Part model, mm, in its own coordinate system. Face numbers are marked on the shaded views. A direction names the side the tool comes from. Round coordinates to 2 decimals unless told otherwise and drop trailing zeros. Loops run counter-clockwise (first coordinate to the right, second up) from the corner with the lowest first, then second, coordinate; pieces in that order, holes last. Notation, with made-up numbers: (33, 40) - (65, 40) arc R23 cw to (65, 76) - close; hole circle Ø5 at (20.5, -15.75). An arc over 180 degrees is marked (long way). Write each question's results on one line, items separated by ' | '. Start each with the question number.
(1) Cut at D-D, the plane x = -32. List the corners of the cut face in (y, z).
(2) Cut at B-B, the plane x = -56. List the corners of the cut face in (y, z).
(3) Flat gauge pins, fed straight in: P1, Ø3, axis at x = -71.55, z = -24.85, coming from the +Y side; P2, Ø2, axis at y = -43.5, z = -5, coming from the +X side; P3, Ø1.5, axis at y = -50.5, z = 24, coming from the +X side; P4, Ø6, axis at x = 71.55, z = -24.85, coming from the +Y side. Where does each tip first touch, or does it go through?
(4) Cut at C-C, the plane z = -17. List the corners of the cut face in (x, y).
(5) Tool access for the marked faces 4, 5, 6 and 7: list every direction of +Z, -Z, +X, -X, +Y, -Y with a clear straight run to the whole face (end or side of a thin tool).
(6) Cut at A-A, the plane x = 31.75. List the corners of the cut face in (y, z), then the cut area to 3 significant figures.
(7) Drill centre lines: L1, parallel to Z at x = 31.75, y = -0.4; L2, parallel to Z at x = -39, y = -20; L3, parallel to Z at x = -31, y = -4.5. Where is each one in solid material? Low to high.
(8) Mould opens along Z. For the marked faces 1, 2 and 3 say: released by +Z, released by -Z, zero draft, split by the parting line, or undercut.
from build123d import *

# Parameters (mm, degrees)
SKETCH1_W             = 171.0436
SKETCH1_H             = 78.613
BOSS_EXTRUDE1_DEPTH   = 58.42
CUT_EXTRUDE1_DEPTH    = 45.72
BOSS_EXTRUDE2_DEPTH   = 7.62
FILLET1_R             = 25.4
F_6_CLEARANCE_HOLE2_D = 3.7973
SKETCH12_R            = 3.302
CUT_EXTRUDE2_DEPTH    = 0.889


with BuildPart() as part:
    # Sketch1 → Boss-Extrude1 (new body)
    with BuildSketch(Plane.XZ):
        with Locations((0, 0.485871825)):
            Rectangle(SKETCH1_W, SKETCH1_H)
        with BuildLine():
            Line((-73.683610441, -1.938038616), (-48.639210441, -26.982438616))
            ThreePointArc((-48.639210441, -26.982438616), (-43.966930256, -30.104356426), (-38.4556, -31.200628175))
            Line((-38.4556, -31.200628175), (38.4556, -31.200628175))
            ThreePointArc((38.4556, -31.200628175), (43.966930256, -30.104356426), (48.639210441, -26.982438616))
            Line((48.639210441, -26.982438616), (73.683610441, -1.938038616))
            ThreePointArc((73.683610441, -1.938038616), (76.805528251, 13.756902081), (63.5, 22.647371825))
            Line((63.5, 22.647371825), (-63.5, 22.647371825))
            ThreePointArc((-63.5, 22.647371825), (-76.805528251, 13.756902081), (-73.683610441, -1.938038616))
        make_face(mode=Mode.SUBTRACT)
    extrude(amount=BOSS_EXTRUDE1_DEPTH)

    # Sketch2 → Cut-Extrude1 (cut)
    with BuildSketch(Plane.XZ.offset(58.42)):
        with BuildLine():
            ThreePointArc((54.027364114, -32.370592289), (46.882978011, -37.144318464), (38.4556, -38.820628175))
            Line((38.4556, -38.820628175), (85.5218, -38.820628175))
            Line((85.5218, -38.820628175), (85.5218, 8.245571825))
            ThreePointArc((85.5218, 8.245571825), (83.845490289, -0.181806186), (79.071764114, -7.326192289))
            Line((79.071764114, -7.326192289), (54.027364114, -32.370592289))
        make_face()
        with BuildLine():
            Line((-85.5218, 8.245571825), (-85.5218, -38.820628175))
            Line((-85.5218, -38.820628175), (-38.4556, -38.820628175))
            ThreePointArc((-38.4556, -38.820628175), (-46.882978011, -37.144318464), (-54.027364114, -32.370592289))
            Line((-54.027364114, -32.370592289), (-79.071764114, -7.326192289))
            ThreePointArc((-79.071764114, -7.326192289), (-83.845490289, -0.181806186), (-85.5218, 8.245571825))
        make_face()
        with BuildLine():
            Line((-85.5218, 39.792371825), (-85.5218, 8.245571825))
            ThreePointArc((-85.5218, 8.245571825), (-79.071764114, 23.817335939), (-63.5, 30.267371825))
            Line((-63.5, 30.267371825), (63.5, 30.267371825))
            ThreePointArc((63.5, 30.267371825), (79.071764114, 23.817335939), (85.5218, 8.245571825))
            Line((85.5218, 8.245571825), (85.5218, 39.792371825))
            Line((85.5218, 39.792371825), (-85.5218, 39.792371825))
        make_face()
    extrude(amount=-CUT_EXTRUDE1_DEPTH, mode=Mode.SUBTRACT)

    # Sketch3 → Boss-Extrude2 (add)
    with BuildSketch(Plane.XZ.offset(58.42)):
        with BuildLine():
            Line((-79.071764114, -7.326192289), (-54.027364114, -32.370592289))
            ThreePointArc((-54.027364114, -32.370592289), (-46.882978011, -37.144318464), (-38.4556, -38.820628175))
            Line((-38.4556, -38.820628175), (38.4556, -38.820628175))
            ThreePointArc((38.4556, -38.820628175), (46.882978011, -37.144318464), (54.027364114, -32.370592289))
            Line((54.027364114, -32.370592289), (79.071764114, -7.326192289))
            ThreePointArc((79.071764114, -7.326192289), (83.845490289, 16.672949836), (63.5, 30.267371825))
            Line((63.5, 30.267371825), (-63.5, 30.267371825))
            ThreePointArc((-63.5, 30.267371825), (-83.845490289, 16.672949836), (-79.071764114, -7.326192289))
        make_face()
    extrude(amount=BOSS_EXTRUDE2_DEPTH)

    # Fillet1
    fillet1_edges = [part.edges().sort_by_distance(p)[0] for p in [
        (85.5218, -6.35, -38.820628175),
        (-85.5218, -6.35, -38.820628175),
        (-85.5218, -6.35, 39.792371825),
        (85.5218, -6.35, 39.792371825),
    ]]
    fillet(fillet1_edges, radius=FILLET1_R)

    # #6 Clearance Hole2 (through all)
    with Locations(Plane(origin=(0, -12.7, 0), x_dir=(-1, 0, 0), z_dir=(0, -1, 0))):
        with Locations((-31.75, -35.029871825), (-71.5518, 24.850628175)):
            f_6_clearance_hole2 = Hole(F_6_CLEARANCE_HOLE2_D / 2)

    # Mirror1: #6 Clearance Hole2 across plane
    add(f_6_clearance_hole2.mirror(Plane(origin=(0, 0, 0), x_dir=(0, 0, 1), z_dir=(1, 0, 0))), mode=Mode.SUBTRACT)

    # Sketch12 → Cut-Extrude2 (cut)
    with BuildSketch(Plane(origin=(0, 0, 0), x_dir=(1, 0, 0), z_dir=(0, 1, 0))):
        with Locations((-71.5518, 24.850628175)):
            Circle(SKETCH12_R)
        with Locations((-31.75, -35.029871825)):
            Circle(SKETCH12_R)
        with Locations((31.75, -35.029871825)):
            Circle(SKETCH12_R)
        with Locations((71.5518, 24.850628175)):
            Circle(SKETCH12_R)
    extrude(amount=-CUT_EXTRUDE2_DEPTH, mode=Mode.SUBTRACT)


solid = part.part
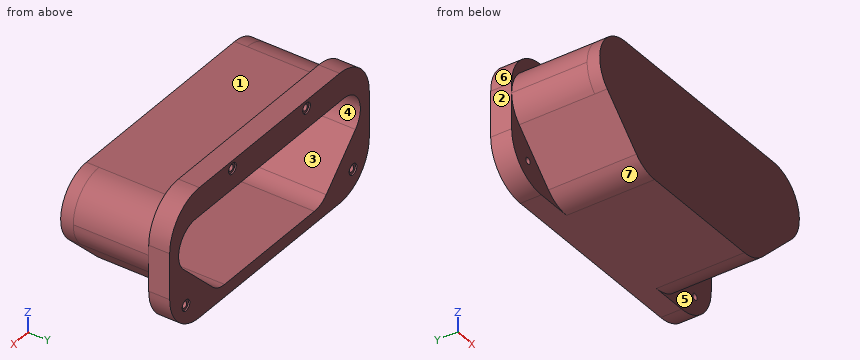
A:
1) outline: (-66.04, -38.82) - (0, -38.82) - (0, -31.2) - (-58.42, -31.2) - (-58.42, 22.65) - (0, 22.65) - (0, 31.74) - (-0.89, 31.74) - (-0.89, 33.15) - (-12.7, 33.15) - (-12.7, 30.27) - (-66.04, 30.27) - close; (-12.7, 36.91) - (-0.89, 36.91) - (-0.89, 38.32) - (0, 38.32) - (0, 39.79) - (-12.7, 39.79) - close
2) outline: (-66.04, -30.4) - (-12.7, -30.4) - (-12.7, -38.82) - (0, -38.82) - (0, -19.62) - (-58.42, -19.62) - (-58.42, 22.65) - (0, 22.65) - (0, 39.79) - (-12.7, 39.79) - (-12.7, 30.27) - (-66.04, 30.27) - close
3) P1: through | P2: x = 81.8 | P3: x = 79.62 | P4: y = -0.89
4) outline: (-85.27, -12.7) - (-69.4, -12.7) - (-69.4, -66.04) - (69.4, -66.04) - (69.4, -12.7) - (85.27, -12.7) - (85.27, 0) - (58.62, 0) - (58.62, -58.42) - (-58.62, -58.42) - (-58.62, 0) - (-85.27, 0) - close
5) face 4: +Y | face 5: -Z, +X, -Y | face 6: +Z, -X, +Y, -Y | face 7: -Z, -X, -Y
6) outline: (-66.04, -38.82) - (0, -38.82) - (0, -31.2) - (-58.42, -31.2) - (-58.42, 22.65) - (0, 22.65) - (0, 31.73) - (-0.89, 31.73) - (-0.89, 33.13) - (-12.7, 33.13) - (-12.7, 30.27) - (-66.04, 30.27) - close; (-12.7, 36.93) - (-0.89, 36.93) - (-0.89, 38.33) - (0, 38.33) - (0, 39.79) - (-12.7, 39.79) - close | area: 1,490 mm2
7) L1: -38.82 to -31.2, 22.65 to 31.73, 38.33 to 39.79 | L2: -38.81 to -31.19, 22.65 to 30.27 | L3: -38.82 to -31.2, 22.65 to 33.29, 36.77 to 39.79
8) face 1: released by +Z | face 2: zero draft | face 3: undercut
